Source: CAD feature listing. Evaluate the final solid. Frame: model axes, mm. A direction names the side the tool comes from. Give positions to 0.01 mm unless a question says otherwise; leave off trailing zeros. Loops run counter-clockwise (first coordinate to the right, second up) from the corner with the lowest first, then second, coordinate; pieces in that order, holes last.
from build123d import *

# Parameters (mm, degrees)
SKETCH1_R                = 30
BOSS_EXTRUDE1_DEPTH      = 10
SKETCH2_R                = 10
BOSS_EXTRUDE2_DEPTH      = 15.25
BOSS_EXTRUDE3_DEPTH      = 13
F_3_0_3_DIAMETER_HOLE1_D = 3
BOSS_EXTRUDE4_DEPTH      = 11
F_4_0_4_DIAMETER_HOLE1_D = 4


with BuildPart() as part:
    # Sketch1 → Boss-Extrude1 (new body)
    with BuildSketch(Plane(origin=(0, 0, 0), x_dir=(1, 0, 0), z_dir=(0, 1, 0))):
        with Locations(Location((0, 0, 0), (0, 0, 270))):
            Circle(SKETCH1_R)
    extrude(amount=BOSS_EXTRUDE1_DEPTH)

    # Sketch2 → Boss-Extrude2 (add)
    with BuildSketch(Plane(origin=(0, 0, 0), x_dir=(-1, 0, 0), z_dir=(0, -1, 0))):
        with Locations(Location((0, 0, 0), (0, 0, 270))):
            Circle(SKETCH2_R)
    extrude(amount=BOSS_EXTRUDE2_DEPTH)

    # Sketch3 → Boss-Extrude3 (add)
    with BuildSketch(Plane(origin=(0, -15.25, 0), x_dir=(-1, 0, 0), z_dir=(0, -1, 0))):
        Polygon((-9, 4), (-9, 0), (-9, -4), (9, -4), (9, 4), align=None)
    extrude(amount=BOSS_EXTRUDE3_DEPTH)

    # Ø3.0 (3) Diameter Hole1 (through all)
    with Locations(Plane.XY.offset(4)):
        with Locations((0, -24.25), (0, -18.25)):
            Hole(F_3_0_3_DIAMETER_HOLE1_D / 2)

    # Sketch8 → Boss-Extrude4 (add)
    with BuildSketch(Plane(origin=(0, 10, 0), x_dir=(1, 0, 0), z_dir=(0, 1, 0))):
        Polygon((-23.1, -7.5), (-23.1, 0), (-23.1, 7.5), (23.1, 7.5), (23.1, -7.5), align=None)
    extrude(amount=BOSS_EXTRUDE4_DEPTH)

    # Ø4.0 (4) Diameter Hole1 (through all)
    with Locations(Plane(origin=(0, 0, -7.5), x_dir=(-1, 0, 0), z_dir=(0, 0, -1))):
        with Locations((-14, 15.5), (14, 15.5)):
            Hole(F_4_0_4_DIAMETER_HOLE1_D / 2)


solid = part.part
1) Pull-direction query (Y, two-part tool) for faces 6 (the flat face through (0, 10, 13)), 7 (the flat face through (0, -28.25, 0)), 8 (the cylindrical face through (0.195, -16.763, -0.056)); classes: released by +Y, released by -Y, zero draft, split by the parting line, or undercut.
Checks:
face 6: released by +Y
face 7: released by -Y
face 8: undercut
2) Cut plane A-A (z = 0). Return loops of the section in (x, y).
Checks:
outline: (-30, 0) - (-10, 0) - (-10, -15.25) - (-9, -15.25) - (-9, -28.25) - (9, -28.25) - (9, -15.25) - (10, -15.25) - (10, 0) - (30, 0) - (30, 10) - (23.1, 10) - (23.1, 21) - (-23.1, 21) - (-23.1, 10) - (-30, 10) - close; hole circle Ø4 at (-14, 15.5); hole circle Ø3 at (0, -24.25); hole circle Ø3 at (0, -18.25); hole circle Ø4 at (14, 15.5)
3) Cut plane B-B (x = 0). Return loops of the section in (y, z).
Checks:
outline: (-28.25, -4) - (-25.75, -4) - (-25.75, 4) - (-28.25, 4) - close; (-22.75, -4) - (-19.75, -4) - (-19.75, 4) - (-22.75, 4) - close; (-16.75, -4) - (-15.25, -4) - (-15.25, -10) - (0, -10) - (0, -30) - (10, -30) - (10, -7.5) - (21, -7.5) - (21, 7.5) - (10, 7.5) - (10, 30) - (0, 30) - (0, 10) - (-15.25, 10) - (-15.25, 4) - (-16.75, 4) - close
4) Ray query, probe 1 along Y at (x, z) = (0, 0); probe 2 along X at (y, z) = (16.5, 2); probe 3 along Y at (x, z) = (-14, -2.5). Return the intervals inside material, ascending.
Checks:
probe 1: y = -28.25 to -25.75, -22.75 to -19.75, -16.75 to 21
probe 2: x = -23.1 to -15.73, -12.27 to 12.27, 15.73 to 23.1
probe 3: y = 0 to 13.5, 17.5 to 21
5) Cut plane C-C (y = -18.25). Return loops of the section in (x, z), and give its area (3 significant figures).
Checks:
outline: (-9, -4) - (-1.5, -4) - (-1.5, 4) - (-9, 4) - close; (1.5, -4) - (9, -4) - (9, 4) - (1.5, 4) - close
area: 120 mm2
6) Contact query for flat-ended pins moving along their axis: P1, Ø2.5, axis at x = 0, y = -18.25, coming from the +Z side; P2, Ø5, axis at x = 10, z = 19.5, coming from the -Y side; P3, Ø10.5, axis at x = -2.5, y = -19, coming from the +Z side; P4, Ø6.5, axis at x = -3.5, y = -22.5, coming from the -Z side. Output: stop coordinate, or through.
Checks:
P1: passes through
P2: stops at y = 0
P3: stops at z = 10
P4: stops at z = -4
7) Cut plane D-D (z = -6.5). Return loops of the section in (x, y).
Checks:
outline: (-29.29, 0) - (-7.6, 0) - (-7.6, -15.25) - (7.6, -15.25) - (7.6, 0) - (29.29, 0) - (29.29, 10) - (23.1, 10) - (23.1, 21) - (-23.1, 21) - (-23.1, 10) - (-29.29, 10) - close; hole circle Ø4 at (-14, 15.5); hole circle Ø4 at (14, 15.5)
8) Reachability of faces 1 (the flat face through (-9, -22, 0)), 2 (the flat face through (0, 15, -7.5)), 3 (the flat face through (0, -22, -4)), 4 (the flat face through (0, -22, 4)), 5 (the flat face through (0, 0, 13)) from +Z, -Z, +X, -X, +Y, -Y: full face, straight path, thin tool, end or side. Return the list, or none.
Checks:
face 1: +Z, -Z, -X, -Y
face 2: -Z, +X, -X, +Y
face 3: -Z, +X, -X, -Y
face 4: +Z, +X, -X, -Y
face 5: -Y
